Here's how the part is built. I have some questions about the finished solid (model axes, mm). Round coordinates to 2 decimals unless told otherwise and drop trailing zeros. Order: outer loops, then holes, each group sorted by start corner. A loop starts at its lowest first (then second) coordinate and runs counter-clockwise, first axis right, second up.
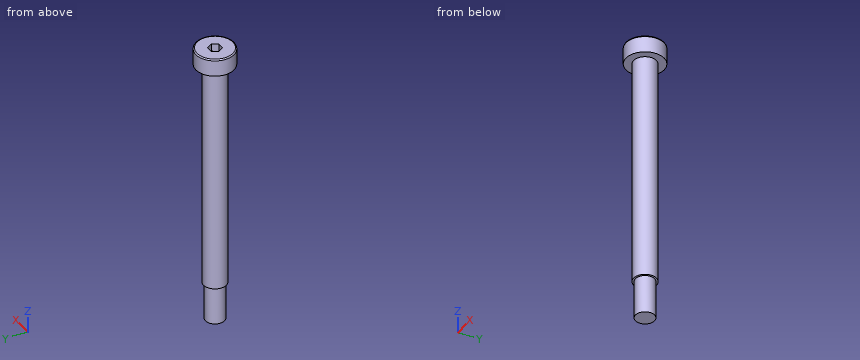
```python
from build123d import *

# Parameters (mm, degrees)
CUT_EXTRUDE_1_DEPTH = 2
FILLET_1_R          = 0.3


with BuildPart() as part:
    # 草图1 → 旋转1 (revolve)
    with BuildSketch(Plane(origin=(0, 0, 0), x_dir=(0, 0, -1), z_dir=(1, 0, 0))):
        Polygon((0, 0), (0, 5), (4.5, 5), (4.5, 3), (64.5, 3), (64.5, 2.5), (74.5, 2.5), (74.5, 0), align=None)
    revolve(axis=Axis((0, 0, -74.5), (0, 0, 1)))

    # 草图2 → 切除-拉伸1 (cut)
    with BuildSketch(Plane.XY):
        Polygon((0.866025404, 1.5), (-0.866025404, 1.5), (-1.732050808, 0), (-0.866025404, -1.5), (0.866025404, -1.5), (1.732050808, 0), align=None)
    extrude(amount=-CUT_EXTRUDE_1_DEPTH, mode=Mode.SUBTRACT)

    # 圆角1
    fillet_1_edges = [part.edges().sort_by_distance(p)[0] for p in [
        (0, -5, 0),
    ]]
    fillet(fillet_1_edges, radius=FILLET_1_R)


solid = part.part
```
1) If we section it at A-A (x = 0): Write out the boundary of the cut face in (y, z).
2) I need wall thicknesses on line 1 (Z direction, x = 0.25, y = 2.75); line 2 (Z direction, x = -1.75, y = -2.5); line 3 (Y direction, x = -0.25, z = -34). Which ranges of each line are inside material? Lowest first, please.
3) If we section it at B-B (z = -50): Write out the boundary of the cut face in (x, y).
4) I'm going to push flat-ended pins straight in: pin 1 (4 mm diameter, centred on x = 0, z = -60.5, fed in from +Y); pin 2 (2 mm diameter, centred on y = -2, z = -55.5, fed in from -X); pin 3 (1.5 mm diameter, centred on x = -2, z = -23, fed in from +Y); pin 4 (3.5 mm diameter, centred on x = 0, y = -0.5, fed in from +Z). Where does each tip first touch, or does it pass through?
Solutions:
1. outline: (-5, -4.5) - (-3, -4.5) - (-3, -64.5) - (-2.5, -64.5) - (-2.5, -74.5) - (2.5, -74.5) - (2.5, -64.5) - (3, -64.5) - (3, -4.5) - (5, -4.5) - (5, -0.3) arc R0.3 ccw to (4.7, 0) - (1.5, 0) - (1.5, -2) - (-1.5, -2) - (-1.5, 0) - (-4.7, 0) arc R0.3 ccw to (-5, -0.3) - close
2. line 1: z = -64.5 to 0
2. line 2: z = -4.5 to 0
2. line 3: y = -2.99 to 2.99
3. outline: circle Ø6 at (0, 0)
4. pin 1: stops at y = 3
4. pin 2: stops at x = -2.83
4. pin 3: stops at y = 2.73
4. pin 4: stops at z = 0
